For this review, take the finished solid that the model builds, in its own axes (mm). Face numbers are marked on the shaded views. A direction names the side the tool comes from. Coordinates: 2 decimals unless noted, no trailing zeros. Loops run counter-clockwise (first coordinate to the right, second up) from the corner with the lowest first, then second, coordinate; pieces in that order, holes last. Notation, with made-up numbers: (-11.5, 44) -> (7.5, 44) arc R10 cw to (7.5, 49) -> close; hole circle Ø8 at (-36, 41.25). An arc over 180 degrees is marked (long way). Use a Markdown table: item, result.
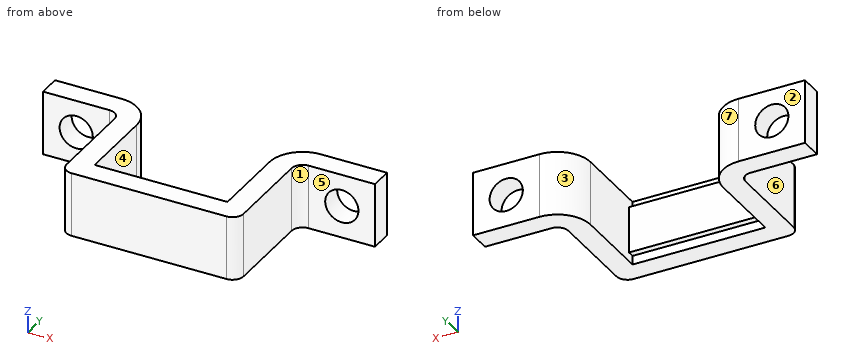
from build123d import *

# Parameters (mm, degrees)
BOSS_EXTRUDE1_DEPTH = 2.9
SKETCH4_W           = 12
SKETCH4_H           = 0.6
BOSS_EXTRUDE2_DEPTH = 2.1
SKETCH5_R           = 1.5
CUT_EXTRUDE1_DEPTH  = 13


with BuildPart() as part:
    # Sketch3 → Boss-Extrude1 (new body, symmetric)
    with BuildSketch(Plane.XY):
        with BuildLine():
            Line((-6, -5), (6, -5))
            Line((6, -5), (6, 2))
            ThreePointArc((6, 2), (6.878679656, 4.121320344), (9, 5))
            Line((9, 5), (15, 5))
            Line((15, 5), (15, 3))
            Line((15, 3), (9, 3))
            ThreePointArc((9, 3), (8.292893219, 2.707106781), (8, 2))
            Line((8, 2), (8, -6))
            ThreePointArc((8, -6), (7.707106781, -6.707106781), (7, -7))
            Line((7, -7), (-7, -7))
            ThreePointArc((-7, -7), (-7.707106781, -6.707106781), (-8, -6))
            Line((-8, -6), (-8, 2))
            ThreePointArc((-8, 2), (-8.292893219, 2.707106781), (-9, 3))
            Line((-9, 3), (-15, 3))
            Line((-15, 3), (-15, 5))
            Line((-15, 5), (-9, 5))
            ThreePointArc((-9, 5), (-6.878679656, 4.121320344), (-6, 2))
            Line((-6, 2), (-6, -5))
        make_face()
    extrude(amount=BOSS_EXTRUDE1_DEPTH, both=True)

    # Sketch4 → Boss-Extrude2 (add, symmetric)
    with BuildSketch(Plane.XY):
        with Locations((0, -4.7)):
            Rectangle(SKETCH4_W, SKETCH4_H)
    extrude(amount=BOSS_EXTRUDE2_DEPTH, both=True)

    # Sketch5 → Cut-Extrude1 (cut, through all)
    with BuildSketch(Plane(origin=(0, 5, 0), x_dir=(1, 0, 0), z_dir=(0, 1, 0))):
        with Locations((12, 0)):
            Circle(SKETCH5_R)
        with Locations((-12, 0)):
            Circle(SKETCH5_R)
    extrude(amount=-CUT_EXTRUDE1_DEPTH, mode=Mode.SUBTRACT)


solid = part.part
(1) For line 1 along Z through (x, y) = (12, 3.4); line 2 along X through (y, z) = (0.75, 2.3); line 3 along X through (y, z) = (4.75, 0.2), list the stretches that pass through material, from the lowest coordinate up.
Found:
| item | result |
|---|---|
| line 1 | z = -2.9 to -1.5, 1.5 to 2.9 |
| line 2 | x = -8 to -6, 6 to 8 |
| line 3 | x = -15 to -13.49, -10.51 to -7.8, 7.8 to 10.51, 13.49 to 15 |
(2) For the marked faces 5, 6 and 7, list the 3-axis set-ups (+Z, -Z, +X, -X, +Y, -Y) from which the entire face can be reached by the end or side of a thin tool; tool diameter is ignored.
Found:
| item | result |
|---|---|
| face 5 | +Z, -Z, +X, -Y |
| face 6 | +Z, -Z, -X, -Y |
| face 7 | +Z, -Z, +Y |
(3) Take a section at A-A on z = 0. Write out the cut boundary in (x, y).
Found:
| item | result |
|---|---|
| outline | (-15, 3) -> (-13.5, 3) -> (-13.5, 5) -> (-15, 5) -> close; (-10.5, 3) -> (-9, 3) arc R1 cw to (-8, 2) -> (-8, -6) arc R1 ccw to (-7, -7) -> (7, -7) arc R1 ccw to (8, -6) -> (8, 2) arc R1 cw to (9, 3) -> (10.5, 3) -> (10.5, 5) -> (9, 5) arc R3 ccw to (6, 2) -> (6, -4.4) -> (-6, -4.4) -> (-6, 2) arc R3 ccw to (-9, 5) -> (-10.5, 5) -> close; (13.5, 3) -> (15, 3) -> (15, 5) -> (13.5, 5) -> close |
(4) For pin 1 Ø3 at (x, z) = (-10.5, -2) entering from -Y; pin 2 Ø3 at (y, z) = (-1.5, -1) entering from -X; pin 3 Ø2 at (x, y) = (-3.5, 1.5) entering from -Z; pin 4 Ø1.5 at (y, z) = (-2, 0) entering from +X, all flat-tipped, find the tip position at first contact; note any pin that passes through.
Found:
| item | result |
|---|---|
| pin 1 | stops at y = 3 |
| pin 2 | stops at x = -8 |
| pin 3 | passes through |
| pin 4 | stops at x = 8 |
(5) Take a section at B-B on x = -12. Write out the cut boundary in (y, z), plus the area to 3 significant figures.
Found:
| item | result |
|---|---|
| outline | (3, -2.9) -> (5, -2.9) -> (5, -1.5) -> (3, -1.5) -> close; (3, 1.5) -> (5, 1.5) -> (5, 2.9) -> (3, 2.9) -> close |
| area | 5.60 mm^2 |
(6) Mouldability with a two-part tool opening along X and no side actions: class the marked faces 1, 2, 3 and 4 as pulls with the +X half, pulls with the -X half, needs draft (parallel to the pull), parting line crosses it, or undercut.
Found:
| item | result |
|---|---|
| face 1 | pulls with the +X half |
| face 2 | needs draft |
| face 3 | undercut |
| face 4 | undercut |
(7) Take a section at D-D on x = 1.75. Write out the cut boundary in (y, z), plus the area to 3 significant figures.
Found:
| item | result |
|---|---|
| outline | (-7, -2.9) -> (-5, -2.9) -> (-5, -2.1) -> (-4.4, -2.1) -> (-4.4, 2.1) -> (-5, 2.1) -> (-5, 2.9) -> (-7, 2.9) -> close |
| area | 14.1 mm^2 |
(8) Take a section at C-C on y = -4. Write out the cut boundary in (x, z).
Found:
| item | result |
|---|---|
| outline | (-8, -2.9) -> (-6, -2.9) -> (-6, 2.9) -> (-8, 2.9) -> close; (6, -2.9) -> (8, -2.9) -> (8, 2.9) -> (6, 2.9) -> close |
